Input: part model. Units: mm. Frame: model coordinates. A direction names the side the tool comes from. Coordinates: 2 decimals unless noted, no trailing zeros. Order: outer loops, then holes, each group sorted by start corner. A loop starts at its lowest first (then second) coordinate and runs counter-clockwise, first axis right, second up. Notation, with made-up numbers: (-19, 31.5) -> (-7, 31.5) arc R25 cw to (-7, 70.5) -> close; hole circle Ø3 at (49.25, -11). An arc over 180 degrees is marked (long way). Use one line per item in the form item = value. Start each with the question number.
1) Section query B-B on x = 4. Output: boundary loops of the cut face in (y, z), then the cut area to 3 significant figures.
2) Pin query (flat end, axial travel): pin 1 (8 mm diameter, centred on y = 14, z = -4.5, fed in from +X); pin 2 (1.5 mm diameter, centred on x = 7, y = 13.5, fed in from -Z); pin 3 (1 mm diameter, centred on x = 4, z = -6, fed in from -Y); pin 4 (5 mm diameter, centred on y = 9, z = -15.5, fed in from -X). Return the tip coordinate at first contact, or that it passes through.
3) Section query A-A on y = -10. Output: boundary loops of the cut face in (x, z).
4) Draft query along Y for faces 1 (the cylindrical face through (2.46, 12.07, -4.35)), 2 (the flat face through (5, 5, -19)), 3 (the flat face through (9, 15, -12)). Return one class per face: pulls with the +Y half, pulls with the -Y half, needs draft (parallel to the pull), parting line crosses it, or undercut.
5) Access query for faces 4 (the flat face through (1, 15, -12)), 5 (the flat face through (5, 0, -10)), 6 (the flat face through (10, 8, -2)), 7 (the flat face through (7.465, 19.31, -7.535)). Directions: +Z, -Z, +X, -X, +Y, -Y. A direction counts if a zero-diameter tool reaches every point of the face in a straight line with its end or side. Return the directions, or none.
6) Section query D-D on z = -17.25. Output: boundary loops of the cut face in (x, y).
7) Ray query, line 1 along Z through (x, y) = (9.5, 15); line 2 along Z through (x, y) = (7, -0.5); line 3 along Y through (x, z) = (5, 3.7). Return the intervals inside material, ascending.
8) Section query C-C on x = 1.5. Output: boundary loops of the cut face in (y, z).
from build123d import *

# Parameters (mm, degrees)
SKETCH_1_R          = 3
EXTRUDE_1_DEPTH     = 5
EXTRUDE_START       = 5
EXTRUDE_2_DEPTH     = 5
SKETCH_3_R          = 2.5
CUT_EXTRUDE_1_DEPTH = 37.742346142
CHAMFER_1_SIZE      = 10
CHAMFER_1_SIZE2     = 5.773502692
SKETCH_4_W          = 8
SKETCH_4_H          = 20
CUT_EXTRUDE_2_DEPTH = 34.541019662
SKETCH_5_R          = 4.5
CUT_EXTRUDE_3_DEPTH = 34.541019662
CUT_EXTRUDE_4_DEPTH = 34.541019662


with BuildPart() as part:
    # 스케치1 → 보스-돌출1 (new body)
    # profile 1 of 2: a face of its own
    with BuildSketch(Plane(origin=(0, 0, 0), x_dir=(0, 0, -1), z_dir=(1, 0, 0))):
        Polygon((20, 0), (0, 0), (0, -20), (-5, -20), (-5, 25), (20, 25), align=None)
        Polygon((10, 17.886751346), (5, 20.773502692), (0, 17.886751346), (0, 12.113248654), (5, 9.226497308), (10, 12.113248654), align=None, mode=Mode.SUBTRACT)
    # profile 2 of 2: a face of its own
    with BuildSketch(Plane(origin=(0, 0, 0), x_dir=(0, 0, -1), z_dir=(1, 0, 0))):
        Polygon((10, 12.113248654), (10, 17.886751346), (5, 20.773502692), (0, 17.886751346), (0, 12.113248654), (5, 9.226497308), align=None)
        with Locations((5, 15)):
            Circle(SKETCH_1_R, mode=Mode.SUBTRACT)
    extrude(amount=EXTRUDE_1_DEPTH)

    # 스케치1<3> → 보스-돌출2 (add)
    with BuildSketch(Plane(origin=(0, 0, 0), x_dir=(0, 0, -1), z_dir=(1, 0, 0)).offset(EXTRUDE_START)):
        Polygon((20, 0), (0, 0), (0, -20), (-5, -20), (-5, 25), (20, 25), align=None)
        Polygon((10, 17.886751346), (5, 20.773502692), (0, 17.886751346), (0, 12.113248654), (5, 9.226497308), (10, 12.113248654), align=None, mode=Mode.SUBTRACT)
    extrude(amount=EXTRUDE_2_DEPTH)

    # 스케치3 → 컷-돌출1 (cut, through all)
    with BuildSketch(Plane.XY.offset(5)):
        with Locations((5, -10)):
            Circle(SKETCH_3_R)
    extrude(amount=-CUT_EXTRUDE_1_DEPTH, mode=Mode.SUBTRACT)

    # 모따기1
    chamfer_1_edges = [part.edges().sort_by_distance(p)[0] for p in [
        (5, 25, 5),
    ]]
    chamfer_1_side = [part.faces().sort_by_distance(p)[0] for p in [
        (5, 25, -7.5),
    ]]
    chamfer(chamfer_1_edges, length=CHAMFER_1_SIZE, length2=CHAMFER_1_SIZE2, reference=chamfer_1_side[0])

    # 스케치4 → 컷-돌출2 (cut, through all)
    with BuildSketch(Plane(origin=(10, 0, 0), x_dir=(0, 0, -1), z_dir=(1, 0, 0))):
        with Locations((16, 15)):
            Rectangle(SKETCH_4_W, SKETCH_4_H)
    extrude(amount=-CUT_EXTRUDE_2_DEPTH, mode=Mode.SUBTRACT)

    # 스케치5 → 컷-돌출3 (cut, through all)
    with BuildSketch(Plane(origin=(0, 5, 0), x_dir=(1, 0, 0), z_dir=(0, 1, 0))):
        with Locations((5, 16)):
            Circle(SKETCH_5_R)
    extrude(amount=CUT_EXTRUDE_3_DEPTH, mode=Mode.SUBTRACT)

    # 스케치5<3> → 컷-돌출4 (cut, through all)
    with BuildSketch(Plane(origin=(0, 5, 0), x_dir=(1, 0, 0), z_dir=(0, 1, 0))):
        with BuildLine():
            ThreePointArc((5, 18.5), (2.5, 16), (5, 13.5))
            Line((5, 13.5), (5, 18.5))
        make_face()
        with BuildLine():
            Line((5, 18.5), (5, 13.5))
            ThreePointArc((5, 13.5), (6.767766953, 14.232233047), (7.5, 16))
            ThreePointArc((7.5, 16), (6.767766953, 17.767766953), (5, 18.5))
        make_face()
    extrude(amount=-CUT_EXTRUDE_4_DEPTH, mode=Mode.SUBTRACT)


solid = part.part
Answers below:
q1.outline = (-20, 0) -> (-12.29, 0) -> (-12.29, 5) -> (-20, 5) -> close; (-7.71, 0) -> (0, 0) -> (0, -13.71) -> (5, -13.71) -> (5, -11.61) -> (25, -11.61) -> (25, -5) -> (19.23, 5) -> (-7.71, 5) -> close; (0, -20) -> (5, -20) -> (5, -18.29) -> (0, -18.29) -> close; hole circle Ø6 at (15, -5)
q1.area = 454 mm^2
q2.pin_1 = 10
q2.pin_2 = -12
q2.pin_3 = 0
q2.pin_4 = through
q3.outline = (0, 0) -> (2.5, 0) -> (2.5, 5) -> (0, 5) -> close; (7.5, 0) -> (10, 0) -> (10, 5) -> (7.5, 5) -> close
q4.face_1 = undercut
q4.face_2 = pulls with the +Y half
q4.face_3 = needs draft
q5.face_4 = -Z, +X, -X, +Y
q5.face_5 = -Z, +X, -X, -Y
q5.face_6 = +Z, -Z, +X, +Y, -Y
q5.face_7 = +X
q6.outline = (0, 0) -> (2.83, 0) -> (2.83, 5) -> (0, 5) -> close; (7.17, 0) -> (10, 0) -> (10, 5) -> (7.17, 5) -> close
q7.line_1 = -12 to -10, 0 to 5
q7.line_2 = 0 to 5
q7.line_3 = -20 to -12.5, -7.5 to 19.98
q8.outline = (-20, 0) -> (0, 0) -> (0, -20) -> (5, -20) -> (5, -12) -> (25, -12) -> (25, -5) -> (19.23, 5) -> (-20, 5) -> close; hole circle Ø6 at (15, -5)
